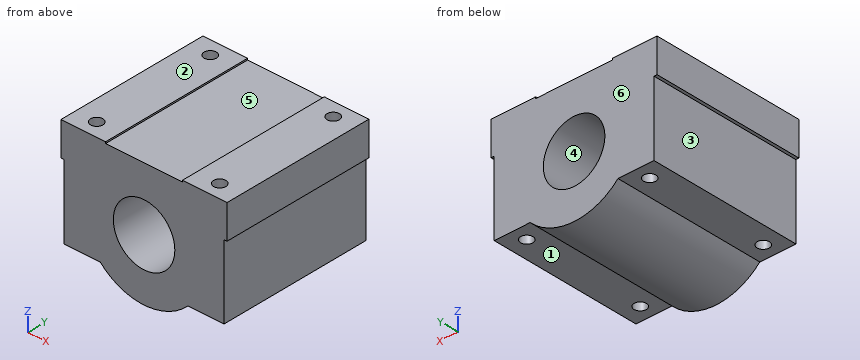
from build123d import *

# Parameters (mm, degrees)
F0_R     = 10
F1_DEPTH = 50
F2_R     = 2
F3_DEPTH = 41.001


with BuildPart() as f1:
    # F0 (on Front) → F1 (new body)
    with BuildSketch(Plane.XZ):
        with BuildLine():
            Line((14.282857, -17.5), (26, -17.5))
            Line((26, -17.5), (26, 6.5))
            Line((26, 6.5), (27, 6.5))
            Line((27, 6.5), (27, 17.5))
            Line((27, 17.5), (12.5, 17.5))
            Line((12.5, 17.5), (12.5, 17))
            Line((12.5, 17), (-12.5, 17))
            Line((-12.5, 17), (-12.5, 17.5))
            Line((-12.5, 17.5), (-27, 17.5))
            Line((-27, 17.5), (-27, 6.5))
            Line((-27, 6.5), (-26, 6.5))
            Line((-26, 6.5), (-26, -17.5))
            Line((-26, -17.5), (-14.282857, -17.5))
            ThreePointArc((-14.282857, -17.5), (0, -23.5), (14.282857, -17.5))
        make_face()
        with Locations((0, -3.5)):
            Circle(F0_R, mode=Mode.SUBTRACT)
    extrude(amount=F1_DEPTH)

    # F2 (on face) → F3 (cut, through all)
    with BuildSketch(Plane.XY.offset(17.5)):
        with Locations((20, -45)):
            Circle(F2_R)
        with Locations((-20, -45)):
            Circle(F2_R)
        with Locations((-20, -5)):
            Circle(F2_R)
        with Locations((20, -5)):
            Circle(F2_R)
    extrude(amount=-F3_DEPTH, mode=Mode.SUBTRACT)


solid = f1.part
For this review, take the finished solid that the model builds, in its own axes (mm). Face numbers are marked on the shaded views. A direction names the side the tool comes from. Give positions to 0.01 mm unless a question says otherwise; leave off trailing zeros. Loops run counter-clockwise (first coordinate to the right, second up) from the corner with the lowest first, then second, coordinate; pieces in that order, holes last. Notation, with made-up numbers: M -30.75,49 L -26.75,49 A24 ccw -26.75,73 Z; hole C 72,2 d5. An arc over 180 degrees is marked long. Answer as a JSON object with one key per item and string values. Group by question number.
Q1. Add section A-A on x = 20. Give the boundary of the cut face in (y, z), and give its area (3 significant figures).
Q2. Add section B-B on z = 2.5. Give the boundary of the cut face in (x, y).
Q3. For probe 1 along Y at (x, z) = (-20, 3.5); probe 2 along X at (y, z) = (-22, -14.5); probe 3 along X at (y, z) = (-22, -3), list the stretches that pass through material, from the lowest coordinate up. Write a range as [from, to].
Q4. Tool access review of the marked faces 1, 2 and 3: name each direction out of +Z, -Z, +X, -X, +Y, -Y from which nothing blocks a thin tool from reaching the whole face with its end or side.
Q5. Add section D-D on x = 0. Give the boundary of the cut face in (y, z).
Q6. Add section C-C on y = -5. Give the boundary of the cut face in (x, z).
Q7. Mouldability with a two-part tool opening along Z and no side actions: class the marked faces 4, 5 and 6 as +Z half, -Z half, draft (parallel to the pull), parting line (faces both ways), or undercut.
Q8. Insertion check: P1, Ø0.8, axis at x = 26.5, y = -14, coming from the -Z side; P2, Ø3.5, axis at x = 19.5, y = -28.5, coming from the -Z side; P3, Ø1.5, axis at y = -40, z = -19, coming from the -X side. Each pin has a flat end and moves straight along its axis. Give the tip position at first contact, or say it passes through.
Checked values:
{
 "1": {"outline": "M -50,-17.5 L -47,-17.5 L -47,17.5 L -50,17.5 Z; M -43,-17.5 L -7,-17.5 L -7,17.5 L -43,17.5 Z; M -3,-17.5 L 0,-17.5 L 0,17.5 L -3,17.5 Z", "area": "1,470 mm²"},
 "2": {"outline": "M -26,-50 L -8,-50 L -8,0 L -26,0 Z; M 8,-50 L 26,-50 L 26,0 L 8,0 Z; hole C -20,-45 d4; hole C -20,-5 d4; hole C 20,-45 d4; hole C 20,-5 d4"},
 "3": {"probe 1": "[-50, -47], [-43, -7], [-3, 0]", "probe 2": "[-26, 26]", "probe 3": "[-26, -9.99], [9.99, 26]"},
 "4": {"face 1": "-Z, +X, +Y, -Y", "face 2": "+Z, +X, -X, +Y, -Y", "face 3": "-Z, -X, +Y, -Y"},
 "5": {"outline": "M -50,-23.5 L 0,-23.5 L 0,-13.5 L -50,-13.5 Z; M -50,6.5 L 0,6.5 L 0,17 L -50,17 Z"},
 "6": {"outline": "M -27,6.5 L -26,6.5 L -26,-17.5 L -22,-17.5 L -22,17.5 L -27,17.5 Z; M -18,-17.5 L -14.28,-17.5 A20 ccw 14.28,-17.5 L 18,-17.5 L 18,17.5 L 12.5,17.5 L 12.5,17 L -12.5,17 L -12.5,17.5 L -18,17.5 Z; M 22,-17.5 L 26,-17.5 L 26,6.5 L 27,6.5 L 27,17.5 L 22,17.5 Z; hole C 0,-3.5 d20"},
 "7": {"face 4": "undercut", "face 5": "+Z half", "face 6": "draft"},
 "8": {"P1": "z = 6.5", "P2": "z = -17.5", "P3": "x = -13.51"}
}
